Geometry: final body of the model. Coordinates: model frame, mm. Give positions to 0.01 mm unless a question says otherwise; leave off trailing zeros. Loops run counter-clockwise (first coordinate to the right, second up) from the corner with the lowest first, then second, coordinate; pieces in that order, holes last. Notation, with made-up numbers: M 26,-1.5 L 51,-1.5 A9 cw 51,7.5 Z; hole C 24,-33 d9. An arc over 180 degrees is marked long. Put each result on its own line as item: value.
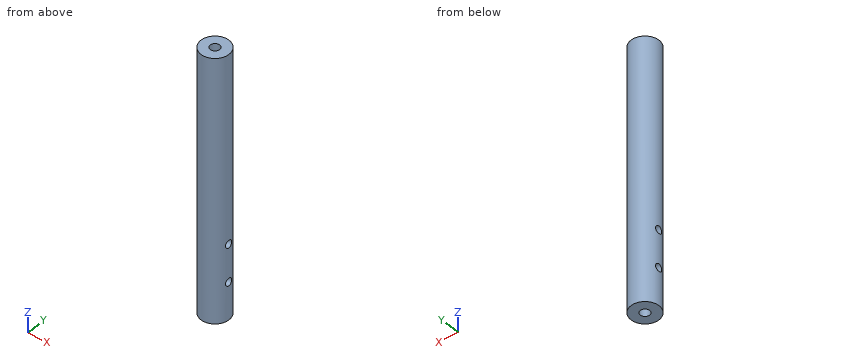
```python
from build123d import *

# Parameters (mm, degrees)
SKETCH1_R           = 7.5
SKETCH1_R_2         = 2.5
BOSS_EXTRUDE1_DEPTH = 140
SKETCH2_R           = 2
CUT_EXTRUDE1_DEPTH  = 16


with BuildPart() as part:
    # Sketch1 → Boss-Extrude1 (new body)
    with BuildSketch(Plane.XY):
        Circle(SKETCH1_R)
        Circle(SKETCH1_R_2, mode=Mode.SUBTRACT)
    extrude(amount=BOSS_EXTRUDE1_DEPTH)

    # Sketch2 → Cut-Extrude1 (cut)
    with BuildSketch(Plane.ZY.offset(7.5)):
        with Locations((20, 0)):
            Circle(SKETCH2_R)
        with Locations((40, 0)):
            Circle(SKETCH2_R)
    extrude(amount=-CUT_EXTRUDE1_DEPTH, mode=Mode.SUBTRACT)


solid = part.part
```
Item 1: Section A-A on x = 0. Output: boundary loops of the cut face in (y, z).
Output values:
outline: M -7.5,0 L -2.5,0 L -2.5,140 L -7.5,140 Z; M 2.5,0 L 7.5,0 L 7.5,140 L 2.5,140 Z
Item 2: Line query: probe 1 along Z at (x, y) = (3, 0); probe 2 along Z at (x, y) = (-5, 0.5); probe 3 along X at (y, z) = (0, 66.5). Output: solid intervals per line, ascending. Write a range as [from, to].
Output values:
probe 1: [0, 18], [22, 38], [42, 140]
probe 2: [0, 18.06], [21.94, 38.06], [41.94, 140]
probe 3: [-7.5, -2.5], [2.5, 7.5]
Item 3: Section C-C on z = 20. Output: boundary loops of the cut face in (x, y).
Output values:
outline: M -7.23,-2 A7.5 ccw 7.23,-2 L 1.5,-2 A2.5 cw -1.5,-2 Z; M -7.23,2 L -1.5,2 A2.5 cw 1.5,2 L 7.23,2 A7.5 ccw Z
Item 4: Pin query (flat end, axial travel): pin 1 Ø2 at (x, y) = (-0.5, -1) entering from +Z; pin 2 Ø5 at (y, z) = (-2.5, 123.5) entering from +X. Return the tip coordinate at first contact, or that it passes through.
Output values:
pin 1: through
pin 2: x = 7.5
Item 5: Section B-B on y = 0. Output: boundary loops of the cut face in (x, z).
Output values:
outline: M -7.5,0 L -2.5,0 L -2.5,18 L -7.5,18 Z; M -7.5,22 L -2.5,22 L -2.5,38 L -7.5,38 Z; M -7.5,42 L -2.5,42 L -2.5,140 L -7.5,140 Z; M 2.5,0 L 7.5,0 L 7.5,18 L 2.5,18 Z; M 2.5,22 L 7.5,22 L 7.5,38 L 2.5,38 Z; M 2.5,42 L 7.5,42 L 7.5,140 L 2.5,140 Z
Item 6: Section D-D on x = -5.25. Output: boundary loops of the cut face in (y, z).
Output values:
outline: M -5.36,0 L 5.36,0 L 5.36,140 L -5.36,140 Z; hole C 0,20 d4; hole C 0,40 d4
